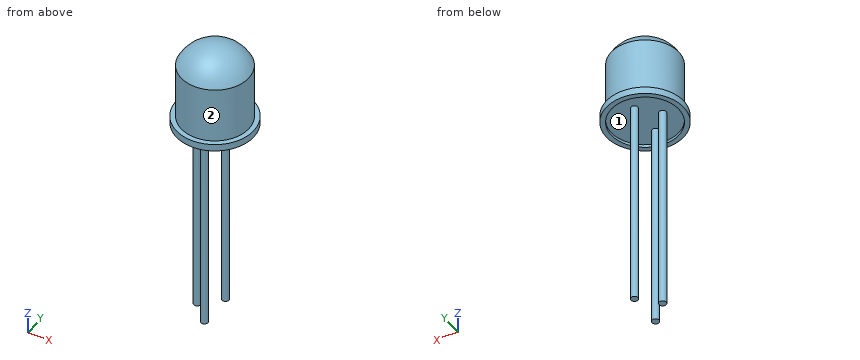
```python
from build123d import *

# Parameters (mm, degrees)
SKETCH2_R           = 2.75
BOSS_EXTRUDE2_DEPTH = 0.5
SKETCH4_R           = 2.4
BOSS_EXTRUDE3_DEPTH = 4
SKETCH5_R           = 2.4
CUT_EXTRUDE1_DEPTH  = 0.2
SKETCH6_R           = 0.25
BOSS_EXTRUDE4_DEPTH = 15


# Read off the part's stored shape, not the designer's step: Dome1
with BuildPart() as part:
    # Sketch2 → Boss-Extrude2 (new body)
    with BuildSketch(Plane.XY):
        Circle(SKETCH2_R)
    extrude(amount=BOSS_EXTRUDE2_DEPTH)

    # Sketch4 → Boss-Extrude3 (add)
    with BuildSketch(Plane.XY.offset(0.5)):
        Circle(SKETCH4_R)
    extrude(amount=BOSS_EXTRUDE3_DEPTH)

    # Dome1 outline → Dome1 (revolve)
    with BuildSketch(Plane.XZ):
        with BuildLine():
            Line((0, 4.5), (2.400000001, 4.499999998))
            ThreePointArc((2.400000001, 4.499999998), (1.415097171, 5.594155471), (0, 6))
            Line((0, 6), (0, 4.5))
        make_face()
    revolve(axis=Axis((0, 0, 0), (0, 0, 1)))

    # Sketch5 → Cut-Extrude1 (cut)
    with BuildSketch(Plane(origin=(0, 0, 0), x_dir=(-1, 0, 0), z_dir=(0, 0, -1))):
        with Locations(Location((0, 0, 0), (0, 0, 180))):
            Circle(SKETCH5_R)
    extrude(amount=-CUT_EXTRUDE1_DEPTH, mode=Mode.SUBTRACT)

    # Sketch6 → Boss-Extrude4 (add)
    with BuildSketch(Plane(origin=(0, 0, 0.2), x_dir=(-1, 0, 0), z_dir=(0, 0, -1))):
        with Locations((0, 1.25)):
            Circle(SKETCH6_R)
        with Locations((1.25, 0)):
            Circle(SKETCH6_R)
        with Locations((0, -1.25)):
            Circle(SKETCH6_R)
    extrude(amount=BOSS_EXTRUDE4_DEPTH)


solid = part.part
```
Design review of the part built by this model. Coordinates are the model's own, in mm. Face numbers are marked on the shaded views. Coordinates: 2 decimals unless noted, no trailing zeros. Loops run counter-clockwise (first coordinate to the right, second up) from the corner with the lowest first, then second, coordinate; pieces in that order, holes last. Notation, with made-up numbers: (0, 76) - (22, 76) arc R14 ccw to (22, 83) - close; hole circle Ø10 at (88.25, 9). An arc over 180 degrees is marked (long way). Use CSV: the item, a comma, the result in double quotes. Start each with the question number.
1) Consider section A-A on x = 0. Write out the cut boundary in (y, z), then the cut area to 3 significant figures.
2) Consider section D-D on x = -1.25. Write out the cut boundary in (y, z), then the cut area to 3 significant figures.
3) The part is to be moulded in two halves that separate along Y. For the marked faces 1 and 2, say which applies: +Y half, -Y half, draft (parallel to the pull), parting line (faces both ways), or undercut.
4) Wall thickness on L1, parallel to Y at x = 0, z = 0.1; L2, parallel to Z at x = -1.85, y = -1.8; L3, parallel to Z at x = -1.5, y = 1.25: over which ranges is each line inside the solid? List them lowest first. Write a range as from..to.
5) Consider section C-C on y = 0. Write out the cut boundary in (x, z).
6) For pin 1 Ø1.6 at (x, y) = (1.5, 1) entering from +Z; pin 2 Ø3 at (x, y) = (0, 0) entering from -Z; pin 3 Ø3 at (y, z) = (-2, -6) entering from +X; pin 4 Ø1 at (x, z) = (1, -1.5) entering from -Y, all flat-tipped, find the tip position at first contact; note any pin that passes through.
7) Consider section B-B on z = -1.25. Write out the cut boundary in (x, y), then the cut area to 3 significant figures.
Geometry says:
1,outline,"(-2.75, 0) - (-2.4, 0) - (-2.4, 0.2) - (-1.5, 0.2) - (-1.5, -14.8) - (-1, -14.8) - (-1, 0.2) - (1, 0.2) - (1, -14.8) - (1.5, -14.8) - (1.5, 0.2) - (2.4, 0.2) - (2.4, 0) - (2.75, 0) - (2.75, 0.5) - (2.4, 0.5) - (2.4, 4.5) arc R2.67 ccw to (-2.4, 4.5) - (-2.4, 0.5) - (-2.75, 0.5) - close"
1,area,"41.1 mm^2"
2,outline,"(-2.45, 0) - (-2.05, 0) - (-2.05, 0.2) - (-0.25, 0.2) - (-0.25, -14.8) - (0.25, -14.8) - (0.25, 0.2) - (2.05, 0.2) - (2.05, 0) - (2.45, 0) - (2.45, 0.5) - (2.05, 0.5) - (2.05, 4.5) arc R2.36 ccw to (-2.05, 4.5) - (-2.05, 0.5) - (-2.45, 0.5) - close"
2,area,"29.0 mm^2"
3,face 1,"undercut"
3,face 2,"parting line"
4,L1,"-2.75..-2.4, -1.5..-1, 1..1.5, 2.4..2.75"
4,L2,"0..0.5"
4,L3,"0.2..5.15"
5,outline,"(-2.75, 0) - (-2.4, 0) - (-2.4, 0.2) - (-1.5, 0.2) - (-1.5, -14.8) - (-1, -14.8) - (-1, 0.2) - (2.4, 0.2) - (2.4, 0) - (2.75, 0) - (2.75, 0.5) - (2.4, 0.5) - (2.4, 4.5) arc R2.67 ccw to (-2.4, 4.5) - (-2.4, 0.5) - (-2.75, 0.5) - close"
6,pin 1,"z = 5.8"
6,pin 2,"z = -14.8"
6,pin 3,"x = 0.25"
6,pin 4,"through"
7,outline,"circle Ø0.5 at (-1.25, 0); circle Ø0.5 at (0, -1.25); circle Ø0.5 at (0, 1.25)"
7,area,"0.589 mm^2"
